Answer from the drawing. Dimensions are ordinates in mm from the lowest x, y and z of the part. Give positions to 0.01 mm unless a question says otherwise; leave off trailing zeros. Write each loop counter-clockwise with the first axis right and the second up, starting at its lowest first coordinate (ties: lowest second). Pieces come first, ordered by that corner, then holes.
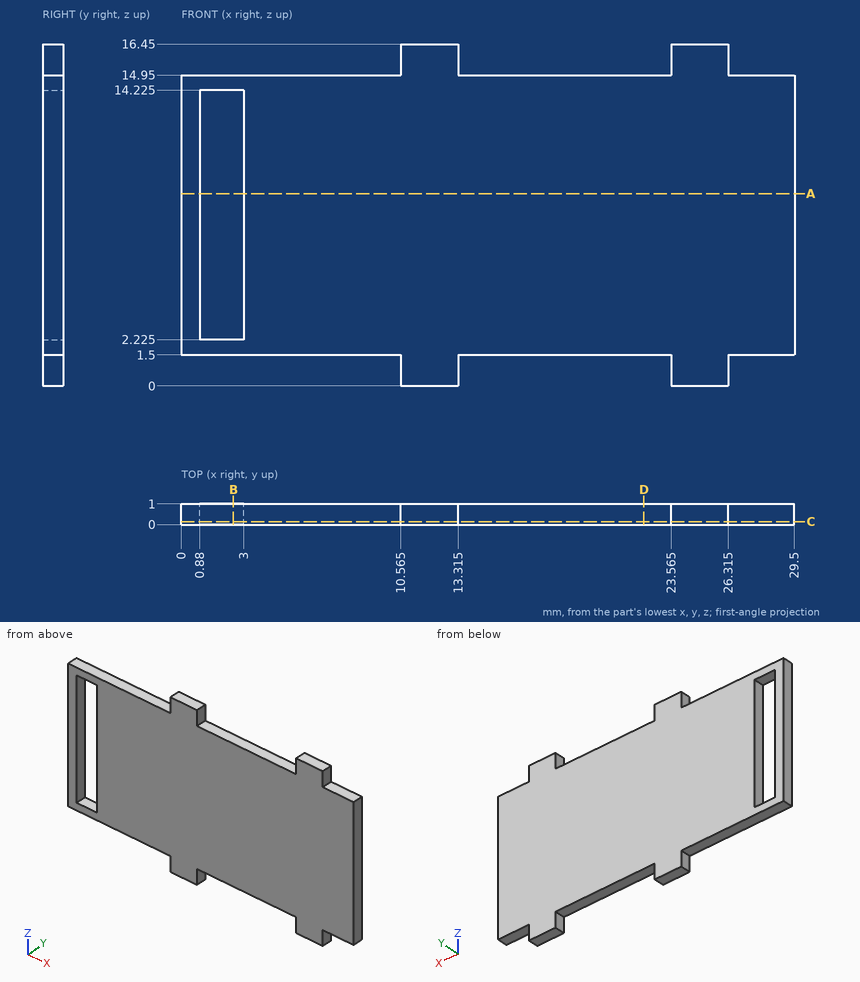
Item 1: A cutting plane is placed at C-C, the plane y = 0.15. Give the vertices of the cut face in (x, z) (3 decimals), plus the area to 3 significant figures.
Conclusion:
outline: (0, 1.5) - (10.565, 1.5) - (10.565, 0) - (13.315, 0) - (13.315, 1.5) - (23.565, 1.5) - (23.565, 0) - (26.315, 0) - (26.315, 1.5) - (29.5, 1.5) - (29.5, 14.95) - (26.315, 14.95) - (26.315, 16.45) - (23.565, 16.45) - (23.565, 14.95) - (13.315, 14.95) - (13.315, 16.45) - (10.565, 16.45) - (10.565, 14.95) - (0, 14.95) - close; hole (0.88, 2.225) - (3, 2.225) - (3, 14.225) - (0.88, 14.225) - close
area: 388 mm2
Item 2: Consider probe 1 along X at (y, z) = (0.2, 6.5); probe 2 along X at (y, z) = (0.6, 16) (3 decimals); probe 3 along Z at (x, y) = (8.5, 0.7). Determine where each line is inside the solid, lowest interval first.
Conclusion:
probe 1: x = 0 to 0.88, 3 to 29.5
probe 2: x = 10.565 to 13.315, 23.565 to 26.315
probe 3: z = 1.5 to 14.95
Item 3: Each of these flat-tipped pins is pushed along its axis until it touches: P1, Ø0.5, axis at y = 0.5, z = 0.5, coming from the -X side (3 decimals); P2, Ø0.5, axis at y = 0.5, z = 1, coming from the +X side (3 decimals); P3, Ø0.5, axis at x = 2.5, y = 0.5, coming from the +Z side. Where does it stop, or does it pass through?
Conclusion:
P1: stops at x = 10.565
P2: stops at x = 26.315
P3: stops at z = 14.95
Item 4: A cutting plane is placed at D-D, the plane x = 22.25. Give the vertices of the cut face in (y, z).
Conclusion:
outline: (0, 1.5) - (1, 1.5) - (1, 14.95) - (0, 14.95) - close
Item 5: A cutting plane is placed at A-A, the plane z = 9.25. Give the vertices of the cut face in (x, y), plus the area to 3 significant figures.
Conclusion:
outline: (0, 0) - (0.88, 0) - (0.88, 1) - (0, 1) - close; (3, 0) - (29.5, 0) - (29.5, 1) - (3, 1) - close
area: 27.4 mm2
Item 6: A cutting plane is placed at B-B, the plane x = 2.5. Give the vertices of the cut face in (y, z) (3 decimals), plus the area to 3 significant figures.
Conclusion:
outline: (0, 1.5) - (1, 1.5) - (1, 2.225) - (0, 2.225) - close; (0, 14.225) - (1, 14.225) - (1, 14.95) - (0, 14.95) - close
area: 1.45 mm2
